Verification items for the finished model (mm, model axes). Face numbers are marked on the shaded views. A direction names the side the tool comes from. Give positions to 0.01 mm unless a question says otherwise; leave off trailing zeros. Loops run counter-clockwise (first coordinate to the right, second up) from the corner with the lowest first, then second, coordinate; pieces in that order, holes last. Notation, with made-up numbers: (-32.75, 41) - (2.25, 41) arc R18 cw to (2.25, 72) - close; hole circle Ø6 at (12, 5.5). An arc over 180 degrees is marked (long way). One line per question, with ' | ' between items. Start each with the question number.
1. Mould release check, pull along X, two halves, no side actions. Record for the marked faces 1, 2 and 3: +X half, -X half, draft (parallel to the pull), parting line (faces both ways), or undercut.
2. Section check A-A, the plane y = 10.5. Enter the section's corners in (x, z) (3 decimals), then the cut area to 3 significant figures.
3. Thickness scan on line 1 along Z through (x, y) = (82.5, 7) (3 decimals); line 2 along Y through (x, z) = (-23, 19.5); line 3 along Y through (x, z) = (36, 19). Record the ranges inside material, lowest first. Write a range as from..to.
4. Depth check by flat-ended pin: pin 1 Ø4 at (y, z) = (-20.5, 64.5) entering from -X (3 decimals); pin 2 Ø1 at (x, z) = (12, 22) entering from -Y; pin 3 Ø4 at (x, z) = (-9, 41.5) entering from +Y. Enter the tip coordinate at first touch or a pass-through.
5. Tool access check on the marked faces 4, 5 and 6. Record the directions out of +Z, -Z, +X, -X, +Y, -Y that give a thin tool (end or side, any length) a straight path to the whole face; none if there is none.
6. Section check B-B, the plane y = -19. Enter the section's corners in (x, z) (3 decimals).
from build123d import *

# Parameters (mm, degrees)
F1_DEPTH = 63.5
F0_W     = 23.437294
F0_H     = 19.05
F0_H_2   = 4.7498
F0_H_3   = 4.7752
F2_DEPTH = 25.4
F3_DEPTH = 7.9375
F5_R     = 6.35


with BuildPart() as f1:
    # F0 (on Front) → F1 (new body, symmetric)
    with BuildSketch(Plane.XZ):
        Polygon((-41.275, -9.525), (41.275, -9.525), (41.275, 9.525), (22.225, 9.525), (-41.275, 9.525), align=None)
    extrude(amount=F1_DEPTH, both=True)

    # F0 (on Front) → F2 (join, symmetric)
    with BuildSketch(Plane.XZ):
        with BuildLine():
            Line((22.225, 9.525), (41.275, 9.525))
            Line((41.275, 9.525), (41.275, 27.854561))
            ThreePointArc((41.275, 27.854561), (44.235343, 37.086423), (52.012294, 42.8752))
            Line((52.012294, 42.8752), (60.325, 42.8752))
            Line((60.325, 42.8752), (60.325, 61.9252))
            Line((60.325, 61.9252), (49.472294, 61.9252))
            ThreePointArc((49.472294, 61.9252), (29.874558, 49.667536), (22.225, 27.854561))
            Line((22.225, 27.854561), (22.225, 9.525))
        make_face()
        with Locations((72.043647, 52.4002)):
            Rectangle(F0_W, F0_H)
        with Locations((72.043647, 64.3001)):
            Rectangle(F0_W, F0_H_2)
        with Locations((72.043647, 40.4876)):
            Rectangle(F0_W, F0_H_3)
    extrude(amount=F2_DEPTH, both=True)

    # F0 (on Front) → F3 (join, symmetric)
    with BuildSketch(Plane.XZ):
        with BuildLine():
            add(Edge.make_bspline(
                [(-41.275, 9.525), (-40.683046, 39.880011), (0, 62.237594), (49.472294, 61.9252)],
                knots=[0, 0, 0, 0, 104.789562, 104.789562, 104.789562, 104.789562], degree=3))
            Line((-41.275, 9.525), (22.225, 9.525))
            Line((22.225, 9.525), (22.225, 27.854561))
            ThreePointArc((22.225, 27.854561), (29.874558, 49.667536), (49.472294, 61.9252))
        make_face()
    extrude(amount=F3_DEPTH, both=True)

    # F0 (on Front) → F4 (revolve)
    with BuildSketch(Plane.XZ):
        Polygon((83.762294, 66.675), (83.762294, 61.9252), (83.762294, 42.8752), (83.762294, 38.1), (111.125, 38.1), (111.125, 66.675), align=None)
    revolve(axis=Axis((83.762294, 0, 52.4002), (0, 0, 1)))

    # F5
    f5_edges = [f1.edges().sort_by_distance(p)[0] for p in [
        (41.275, -63.5, 0),
        (41.275, 63.5, 0),
        (-41.275, 63.5, 0),
        (-41.275, -63.5, 0),
    ]]
    fillet(f5_edges, radius=F5_R)


solid = f1.part
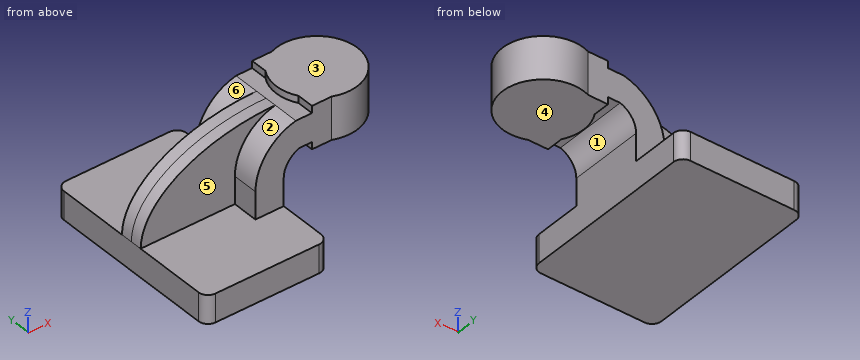
Results list:
1) face 1: undercut | face 2: -X half | face 3: draft
2) outline: (-41.275, -9.525) - (41.275, -9.525) - (41.275, 27.855) arc R15.875 cw to (52.012, 42.875) - (58.494, 42.875) - (58.494, 38.1) - (109.03, 38.1) - (109.03, 66.675) - (58.494, 66.675) - (58.494, 61.925) - (49.472, 61.925) arc R34.925 ccw to (22.225, 27.855) - (22.225, 9.525) - (-41.275, 9.525) - close | area: 4,150 mm²
3) line 1: 38.1..66.675 | line 2: -7.94..7.94 | line 3: -25.4..25.4
4) pin 1: x = 60.325 | pin 2: y = -7.94 | pin 3: y = 7.94
5) face 4: -Z, +X, +Y, -Y | face 5: +Z, -X, -Y | face 6: +Z, -X, +Y
6) outline: (-41.275, -9.525) - (41.275, -9.525) - (41.275, 27.855) arc R15.875 cw to (52.012, 42.875) - (60.325, 42.875) - (60.325, 38.1) - (103.453, 38.1) - (103.453, 66.675) - (60.325, 66.675) - (60.325, 61.925) - (49.472, 61.925) arc R34.925 ccw to (22.225, 27.855) - (22.225, 9.525) - (-41.275, 9.525) - close
